Autodesk Inventor part; units mm, degrees
ref_plane "YZ Plane" through (0, 0, 0) normal (1, 0, 0) x (0, 1, 0)
ref_plane "XZ Plane" through (0, 0, 0) normal (0, 1, 0) x (-1, 0, 0)
ref_plane "XY Plane" through (0, 0, 0) normal (0, 0, 1) x (1, 0, 0)
sketch "Sketch1" plane through (0, 0, 0) normal (0, 1, 0) x (-1, 0, 0)
  line L0 (-231, 355.6) -> (231, 355.6)
  line L1 (231, 355.6) -> (231, -355.6)
  line L2 (231, -355.6) -> (-231, -355.6)
  line L3 (-231, -355.6) -> (-231, 355.6)
  line L4 (-231, 355.6) -> (231, -355.6) construction
  line L5 (231, 355.6) -> (-231, -355.6) construction
  point P0 (0, 0)
  dimension "d0" = 462
  dimension "d1" = 711.2
extrude "Extrusion1" add sketch "Sketch1" along normal blind 19.05
fillet "Fillet1" radius 38.1 4 edges at (231, 9.525, 355.6) (-231, 9.525, 355.6) (-231, 9.525, -355.6) (231, 9.525, -355.6)
sketch "Sketch2" plane through (0, 19.05, 0) normal (0, 1, 0) x (1, 0, 0)
  line L0 (152.8766, -178.8891) -> (-179.8029, -178.8891) construction
  line L1 (-179.8029, -178.8891) -> (-179.8029, 264.6836) construction
  line L2 (-179.8029, 264.6836) -> (152.8766, 264.6836) construction
  line L3 (152.8766, 264.6836) -> (152.8766, -178.8891) construction
  line L4 (0, -29.5589) -> (0, 30.9666) construction
  line L5 (0, 30.9666) -> (0, 0.7039) construction
  line L6 (97.858, 0) -> (-105.142, 0) construction
  point P0 (0, 0)
  dimension "d23" = 203
  dimension "d28" = 60.5255
  dimension "d29" = 178.8891
  dimension "d31" = 55.0186
  dimension "d32" = 152.8766
  dimension "d34" = 149.3302
  dimension "d41" = 332.6795
sketch "Sketch3" plane through (0, 19.05, 0) normal (0, 1, 0) x (1, 0, 0)
  circle A0 centre (-177.8454, 303.3116) radius 27.0466
  point P0 (0, 0)
extrude "Extrusion2" cut sketch "Sketch3" against normal blind 1
sketch "Sketch4" plane through (0, 19.05, 0) normal (0, 1, 0) x (1, 0, 0)
  point P0 (0, 0)
sketch "Sketch5" plane through (0, 19.05, 0) normal (0, 1, 0) x (1, 0, 0)
  line L0 (-102.322, -272.8587) -> (120.5938, -272.8587) construction
  line L1 (120.5938, -272.8587) -> (120.5938, -330.1103) construction
  line L2 (120.5938, -330.1103) -> (-102.322, -330.1103) construction
  line L3 (-102.322, -330.1103) -> (-102.322, -272.8587) construction
  line L4 (-129.111, -331.4845) -> (-129.111, -271.4845)
  line L5 (-129.111, -271.4845) -> (-87.9068, -271.4845)
  line L6 (-87.9068, -271.4845) -> (-87.9068, -281.6369)
  line L7 (-87.9068, -281.6369) -> (-116.9921, -281.6369)
  line L8 (-116.9921, -281.6369) -> (-116.9921, -295.8137)
  line L9 (-116.9921, -295.8137) -> (-91.8854, -295.8137)
  line L10 (-91.8854, -295.8137) -> (-91.8854, -305.9662)
  line L11 (-91.8854, -305.9662) -> (-116.9921, -305.9662)
  line L12 (-116.9921, -305.9662) -> (-116.9921, -331.4845)
  line L13 (-116.9921, -331.4845) -> (-129.111, -331.4845)
  line L14 (-77.8915, -331.4845) -> (-77.8915, -271.4845)
  line L15 (-77.8915, -271.4845) -> (-52.3732, -271.4845)
  spline S0 degree 2 poles (-52.3732, -271.4845) (-42.7239, -271.4845) (-34.0348, -274.7314) (-28.7757, -282.9631) (-28.7757, -288.3137) knots 0 0 0 1 2 3 3 3
  spline S1 degree 2 poles (-28.7757, -288.3137) (-28.7757, -295.0363) (-36.6873, -303.8625) (-44.5989, -305.0058) knots 0 0 0 1 2 2 2
  spline S2 degree 2 poles (-44.5989, -305.0058) (-40.6659, -307.2924) (-35.544, -312.7802) (-31.1995, -319.7771) knots 0 0 0 1 2 2 2
  line L16 (-31.1995, -319.7771) -> (-23.8824, -331.4845)
  line L17 (-23.8824, -331.4845) -> (-38.3793, -331.4845)
  line L18 (-38.3793, -331.4845) -> (-47.1141, -318.4052)
  spline S3 degree 2 poles (-47.1141, -318.4052) (-51.8245, -311.4082) (-55.2543, -307.7497) (-59.0958, -306.4235) (-63.3031, -306.4235) knots 0 0 0 1 2 3 3 3
  line L19 (-63.3031, -306.4235) -> (-65.7726, -306.4235)
  line L20 (-65.7726, -306.4235) -> (-65.7726, -331.4845)
  line L21 (-65.7726, -331.4845) -> (-77.8915, -331.4845)
  line L22 (-65.7726, -296.8656) -> (-56.8092, -296.8656)
  spline S4 degree 2 poles (-56.8092, -296.8656) (-48.0745, -296.8656) (-43.73, -295.4021) (-41.2604, -291.7893) (-41.2604, -289.0912) knots 0 0 0 1 2 3 3 3
  spline S5 degree 2 poles (-41.2604, -289.0912) (-41.2604, -286.0729) (-44.5074, -282.3229) (-47.4342, -281.8198) knots 0 0 0 1 2 2 2
  spline S6 degree 2 poles (-47.4342, -281.8198) (-48.9434, -281.6369) (-56.3062, -281.6369) knots 0 0 0 1 1 1
  line L23 (-56.3062, -281.6369) -> (-65.7726, -281.6369)
  line L24 (-65.7726, -281.6369) -> (-65.7726, -296.8656)
  spline S7 degree 2 poles (-19.8123, -301.8503) (-19.8123, -292.704) (-17.0684, -286.4845) knots 0 0 0 1 1 1
  spline S8 degree 2 poles (-17.0684, -286.4845) (-15.0104, -281.9113) (-7.922, -274.5942) (-3.7147, -272.8564) knots 0 0 0 1 2 2 2
  spline S9 degree 2 poles (-3.7147, -272.8564) (1.8646, -270.4784) (9.2274, -270.4784) knots 0 0 0 1 1 1
  spline S10 degree 2 poles (9.2274, -270.4784) (22.4896, -270.4784) (38.4042, -286.9418) (38.4042, -301.5759) knots 0 0 0 1 2 2 2
  spline S11 degree 2 poles (38.4042, -301.5759) (38.4042, -316.0729) (22.581, -332.4906) (9.3646, -332.4906) knots 0 0 0 1 2 2 2
  spline S12 degree 2 poles (9.3646, -332.4906) (-3.9891, -332.4906) (-19.8123, -316.1643) (-19.8123, -301.8503) knots 0 0 0 1 2 2 2
  spline S13 degree 2 poles (-7.3275, -301.4387) (-7.3275, -311.6369) (2.0932, -322.1552) (9.3646, -322.1552) knots 0 0 0 1 2 2 2
  spline S14 degree 2 poles (9.3646, -322.1552) (16.6359, -322.1552) (25.9194, -311.7284) (25.9194, -301.3015) knots 0 0 0 1 2 2 2
  spline S15 degree 2 poles (25.9194, -301.3015) (25.9194, -290.9662) (16.8646, -280.8137) (9.3646, -280.8137) knots 0 0 0 1 2 2 2
  spline S16 degree 2 poles (9.3646, -280.8137) (1.8646, -280.8137) (-7.3275, -291.1034) (-7.3275, -301.4387) knots 0 0 0 1 2 2 2
  line L25 (47.9621, -331.4845) -> (47.9621, -271.4845)
  line L26 (47.9621, -271.4845) -> (59.7152, -271.4845)
  line L27 (59.7152, -271.4845) -> (84.3646, -311.7284)
  line L28 (84.3646, -311.7284) -> (84.3646, -271.4845)
  line L29 (84.3646, -271.4845) -> (95.5688, -271.4845)
  line L30 (95.5688, -271.4845) -> (95.5688, -331.4845)
  line L31 (95.5688, -331.4845) -> (83.4499, -331.4845)
  line L32 (83.4499, -331.4845) -> (59.1664, -292.1095)
  line L33 (59.1664, -292.1095) -> (59.1664, -331.4845)
  line L34 (59.1664, -331.4845) -> (47.9621, -331.4845)
  line L35 (121.9103, -331.4845) -> (121.9103, -281.6369)
  line L36 (121.9103, -281.6369) -> (104.1207, -281.6369)
  line L37 (104.1207, -281.6369) -> (104.1207, -271.4845)
  line L38 (104.1207, -271.4845) -> (151.7731, -271.4845)
  line L39 (151.7731, -271.4845) -> (151.7731, -281.6369)
  line L40 (151.7731, -281.6369) -> (134.0292, -281.6369)
  line L41 (134.0292, -281.6369) -> (134.0292, -331.4845)
  line L42 (134.0292, -331.4845) -> (121.9103, -331.4845)
  point P0 (0, 0)
extrude "Extrusion3" cut sketch "Sketch5" against normal blind 1
sketch "Sketch6" plane through (0, 19.05, 0) normal (0, 1, 0) x (1, 0, 0)
  line L0 (4.2298, -29.5589) -> (-21.0762, -29.5589)
  line L1 (12.3982, 30.9666) -> (-3.642, 30.9666)
  line L2 (82.3546, 64.3536) -> (37.925, 37.9738)
  line L3 (-29.9268, 38.433) -> (-86.7171, 73.5282)
  line L4 (-49.372, -38.3358) -> (-89.4828, -65.8681)
  line L5 (34.0297, -39.4096) -> (80.2832, -73.7401)
  line L6 (0, -29.5589) -> (0, 30.9666) construction
  line L7 (97.858, 0) -> (-105.142, 0) construction
  arc A0 (-21.0762, -29.5589) -> (-49.372, -38.3358) centre (-21.0762, -79.5589) ccw
  arc A1 (34.0297, -39.4096) -> (4.2298, -29.5589) centre (4.2298, -79.5589) ccw
  arc A2 (12.3982, 30.9666) -> (37.925, 37.9738) centre (12.3982, 80.9666) ccw
  arc A3 (-29.9268, 38.433) -> (-3.642, 30.9666) centre (-3.642, 80.9666) ccw
  arc A4 (97.4597, 55.8264) -> (82.3546, 64.3536) centre (87.4599, 55.7551) ccw
  arc A5 (80.2832, -73.7401) -> (97.0614, -65.4261) centre (86.549, -65.2981) ccw
  arc A6 (-105.142, -57.6234) -> (-89.4828, -65.8681) centre (-95.142, -57.6234) ccw
  arc A7 (-86.7171, 73.5282) -> (-101.9624, 65.5063) centre (-91.9741, 65.0214) ccw
  line L8 (-101.9624, 65.5063) -> (-105.142, 0)
  line L9 (-105.142, -57.6234) -> (-105.142, 0)
  line L10 (97.0614, -65.4261) -> (97.858, 0)
  line L11 (97.4597, 55.8264) -> (97.858, 0)
  point P0 (0, 0)
  dimension "d56" = 50
  dimension "d57" = 50
  dimension "d58" = 50
  dimension "d59" = 10
  dimension "d61" = 10
  dimension "d62" = 10
extrude "Extrusion4" cut sketch "Sketch6" against normal through all
sketch "Sketch7" plane through (0, 19.05, 0) normal (0, 1, 0) x (1, 0, 0)
  circle A0 centre (121.5557, -81.9528) radius 4.2334
  circle A1 centre (124.4127, 77.4269) radius 4.3443
  circle A2 centre (-119.85, 82.8926) radius 4.0735
  circle A3 centre (-124.0139, -75.9442) radius 4.2163
  point P0 (0, 0)
extrude "Extrusion5" cut sketch "Sketch7" against normal blind 1
equation "\"d57\" = d56"
equation "\"d58\" = d57"
properties part number "BaseBoard"
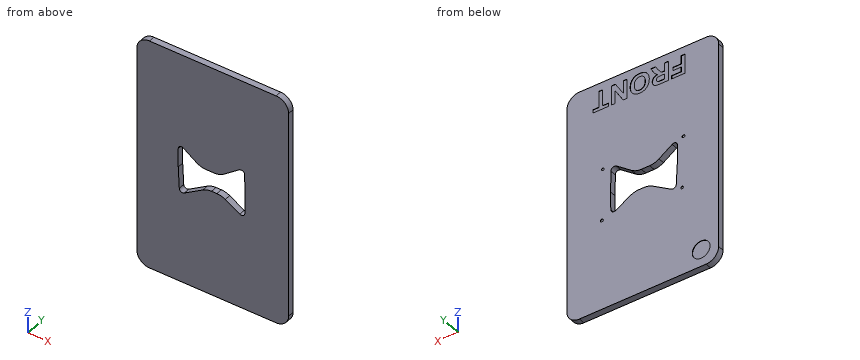
Input: part model. Units: mm. Frame: model coordinates. Coordinates: 2 decimals unless noted, no trailing zeros. Order: outer loops, then holes, each group sorted by start corner. A loop starts at its lowest first (then second) coordinate and runs counter-clockwise, first axis right, second up.
1. Cut plane A-A, the plane z = 12. Return loops of the section in (x, y).
Checked values:
outline: (-231, 0) - (-105.14, 0) - (-105.14, 19.05) - (-231, 19.05) - close; (97.71, 0) - (231, 0) - (231, 19.05) - (97.71, 19.05) - close
2. Contact query for flat-ended pins moving along their axis: P1, Ø0.8, axis at y = 18.5, z = 319.5, coming from the -X side; P2, Ø4, axis at x = -119.5, z = -84, coming from the +Y side. Output: stop coordinate, or through.
Checked values:
P1: stops at x = -230.97
P2: stops at y = 18.05
3. Cut plane B-B, the plane y = 6.25. Return loops of the section in (x, z) (3 decimals), plus the area to 3 significant figures.
Checked values:
outline: (-231, -317.5) arc R38.1 ccw to (-192.9, -355.6) - (192.9, -355.6) arc R38.1 ccw to (231, -317.5) - (231, 317.5) arc R38.1 ccw to (192.9, 355.6) - (-192.9, 355.6) arc R38.1 ccw to (-231, 317.5) - close; hole (-105.142, 0) - (-101.962, -65.506) arc R10 ccw to (-86.717, -73.528) - (-29.927, -38.433) arc R50 cw to (-3.642, -30.967) - (12.398, -30.967) arc R50 cw to (37.925, -37.974) - (82.355, -64.354) arc R10 ccw to (97.46, -55.826) - (97.858, 0) - (97.061, 65.426) arc R10.513 ccw to (80.283, 73.74) - (34.03, 39.41) arc R50 cw to (4.23, 29.559) - (-21.076, 29.559) arc R50 cw to (-49.372, 38.336) - (-89.483, 65.868) arc R10 ccw to (-105.142, 57.623) - close
area: 308,000 mm2
4. Ray query, line 1 along Z through (x, y) = (3, 10.25); line 2 along X through (y, z) = (1, -69); line 3 along X through (y, z) = (11, 62). Return the intervals inside material, ascending.
Checked values:
line 1: z = -355.6 to -30.97, 29.56 to 355.6
line 2: x = -231 to -101.15, -79.39 to 231
line 3: x = -231 to -104.13, -83.85 to 64.47, 97.1 to 231
